Autodesk Inventor part; units mm, degrees
ref_plane "YZ Plane" through (0, 0, 0) normal (1, 0, 0) x (0, 1, 0)
ref_plane "XZ Plane" through (0, 0, 0) normal (0, 1, 0) x (-1, 0, 0)
ref_plane "XY Plane" through (0, 0, 0) normal (0, 0, 1) x (1, 0, 0)
sketch "スケッチ1" plane through (0, 0, 0) normal (0, 0, 1) x (1, 0, 0)
  line L0 (0, 0) -> (100, 0)
  line L1 (100, 0) -> (100, 180)
  line L2 (100, 180) -> (0, 180)
  line L3 (0, 180) -> (0, 0)
  line L4 (0, 10) -> (100, 10) construction
  circle A0 centre (10, 10) radius 2.5
  circle A1 centre (90, 10) radius 2.5
  circle A2 centre (10, 130) radius 5
  circle A3 centre (10, 50) radius 5
  circle A4 centre (90, 130) radius 5
  circle A5 centre (90, 50) radius 5
  line L5 (10, 130) -> (10, 50) construction
  line L6 (10, 50) -> (90, 50) construction
  line L7 (90, 50) -> (90, 130) construction
  line L8 (90, 130) -> (10, 130) construction
  line L9 (0, 90) -> (100, 90) construction
  circle A6 centre (10, 170) radius 2.5
  circle A7 centre (90, 170) radius 2.5
  dimension "d0" = 5
  dimension "d1" = 10
  dimension "d2" = 10
  dimension "d3" = 10
  dimension "d4" = 100
  dimension "d5" = 180
  dimension "d12" = 10
  dimension "d13" = 10
  dimension "d15" = 10
  dimension "d21" = 80
  dimension "d23" = 50
extrude "押し出し1" add sketch "スケッチ1" along normal blind 3
fillet "フィレット1" radius 5 4 edges at (100, 180, 1.5) (0, 180, 1.5) (100, 0, 1.5) (0, 0, 1.5)
properties part number "LRFマウント"
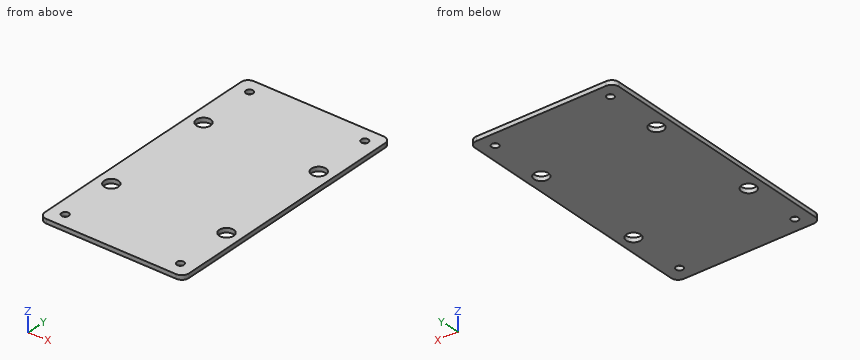
The listing builds one solid part. Answer for the finished solid, in the listing's coordinates (mm). Round coordinates to 2 decimals unless told otherwise and drop trailing zeros. Order: outer loops, then holes, each group sorted by start corner. A loop starts at its lowest first (then second) coordinate and runs counter-clockwise, first axis right, second up. Notation, with made-up numbers: (39, 27.5) - (91, 27.5) arc R4 ccw to (91, 31.5) - close; hole circle Ø11 at (51, 52). An arc over 180 degrees is marked (long way). Put each result on its own line as item: value. Start each with the question number.
(1) Given P1, Ø8, axis at x = 10, y = 130, coming from the +Z side, flat-ended and moving along its own axis, determine where the tip first touches the part or whether it passes through.
(2) Find section C-C (x = 10). Give the vertices of the cut face in (y, z).
(3) Straight lines are drawn through the part: probe 1 along Y at (x, z) = (10, 2.25); probe 2 along X at (y, z) = (170, 0.7); probe 3 along Y at (x, z) = (90.5, 1.05). For each, find the intervals that lie inside material, in ascending order. Write a range as from..to.
(4) Find section A-A (z = 1.75). State how many separate pieces and enclosed holes the cut face has, plus the area to 3 significant figures.
(5) Find section D-D (y = 130). Give the vertices of the cut face in (x, z).
(6) Find section B-B (y = 170). Give the vertices of the cut face in (x, z), plus the area to 3 significant figures.
Reply:
1. P1: through
2. outline: (0, 0) - (7.5, 0) - (7.5, 3) - (0, 3) - close; (12.5, 0) - (45, 0) - (45, 3) - (12.5, 3) - close; (55, 0) - (125, 0) - (125, 3) - (55, 3) - close; (135, 0) - (167.5, 0) - (167.5, 3) - (135, 3) - close; (172.5, 0) - (180, 0) - (180, 3) - (172.5, 3) - close
3. probe 1: 0..7.5, 12.5..45, 55..125, 135..167.5, 172.5..180
3. probe 2: 0..7.5, 12.5..87.5, 92.5..100
3. probe 3: 0..7.55, 12.45..45.03, 54.97..125.03, 134.97..167.55, 172.45..180
4. separate pieces: 1
4. enclosed holes: 8
4. area: 17,600 mm^2
5. outline: (0, 0) - (5, 0) - (5, 3) - (0, 3) - close; (15, 0) - (85, 0) - (85, 3) - (15, 3) - close; (95, 0) - (100, 0) - (100, 3) - (95, 3) - close
6. outline: (0, 0) - (7.5, 0) - (7.5, 3) - (0, 3) - close; (12.5, 0) - (87.5, 0) - (87.5, 3) - (12.5, 3) - close; (92.5, 0) - (100, 0) - (100, 3) - (92.5, 3) - close
6. area: 270 mm^2
